Job drawing, mm, ordinate dimensions from the low corner. One solid piece. Give positions to 0.01 mm unless a question says otherwise; leave off trailing zeros. Order: outer loops, then holes, each group sorted by start corner. A loop starts at its lowest first (then second) coordinate and runs counter-clockwise, first axis right, second up. Notation, with made-up numbers: (6, 67) -> (13, 67) arc R9 ccw to (13, 75) -> close; hole circle Ø10 at (88, 29). An arc over 180 degrees is marked (long way). Use CSV: the item, a comma, the result in double quotes. Start each with the question number.
1. Cut at B-B on z = 63.5. List the corners of the cut face in (x, y) (3 decimals).
2. Cut at A-A on x = 63.5. List the corners of the cut face in (y, z) (3 decimals), then the cut area to 3 significant figures.
3. Cut at D-D on y = 1.55. List the corners of the cut face in (x, z) (3 decimals), then the cut area to 3 significant figures.
4. Drop a flat-ended pin along its axis: pin 1 (2.5 mm diameter, centred on x = 44.45, z = 31.75, fed in from +Y). Give the stop position or say it passes through.
5. Wall check: line 1 (X direction, y = 2.05, z = 95.25) (3 decimals); line 2 (Z direction, x = 76.5, y = 1.5); line 3 (Z direction, x = 71, y = 1). Give the ranges that are in metal, low to high. Write a range as from..to.
6. Cut at C-C on z = 95.25. List the corners of the cut face in (x, y) (3 decimals), then the cut area to 3 significant figures.
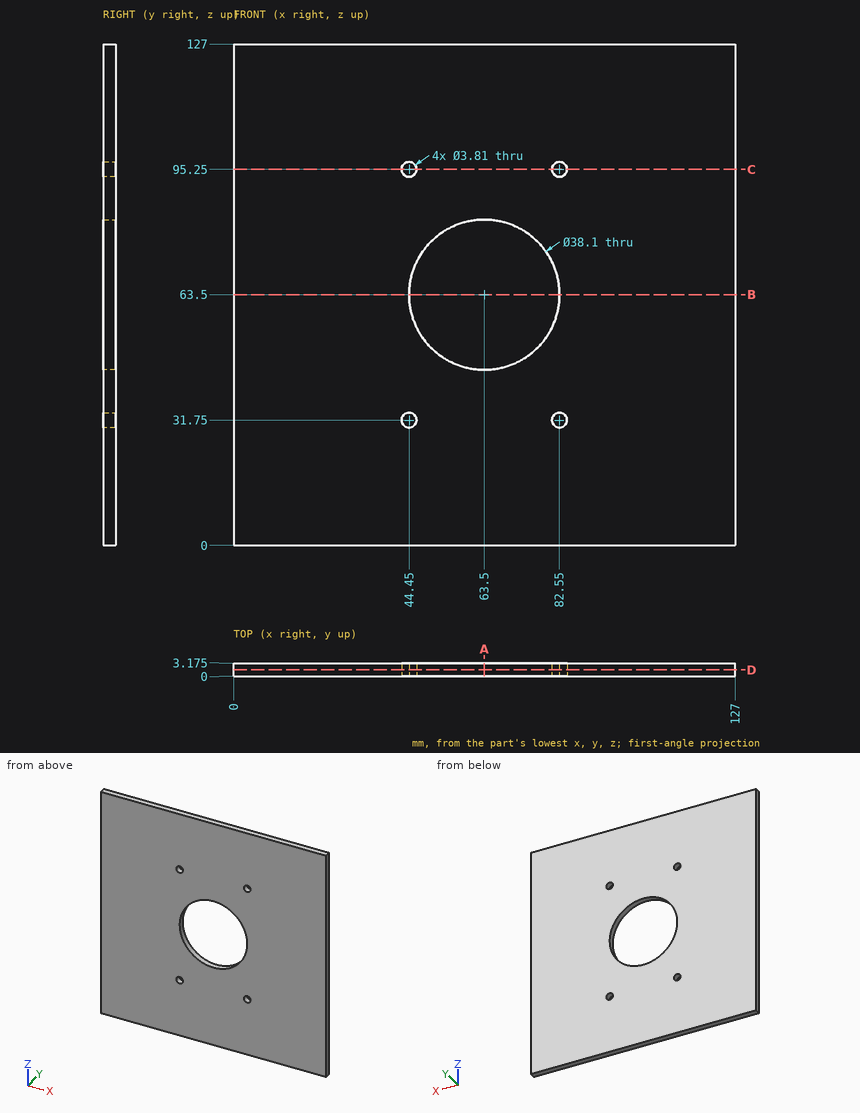
Verdict:
1,outline,"(0, 0) -> (44.45, 0) -> (44.45, 3.175) -> (0, 3.175) -> close; (82.55, 0) -> (127, 0) -> (127, 3.175) -> (82.55, 3.175) -> close"
2,outline,"(0, 0) -> (3.175, 0) -> (3.175, 44.45) -> (0, 44.45) -> close; (0, 82.55) -> (3.175, 82.55) -> (3.175, 127) -> (0, 127) -> close"
2,area,"282 mm^2"
3,outline,"(0, 0) -> (127, 0) -> (127, 127) -> (0, 127) -> close; hole circle Ø3.81 at (44.45, 31.75); hole circle Ø3.81 at (44.45, 95.25); hole circle Ø38.1 at (63.5, 63.5); hole circle Ø3.81 at (82.55, 31.75); hole circle Ø3.81 at (82.55, 95.25)"
3,area,"14,900 mm^2"
4,pin 1,"through"
5,line 1,"0..42.545, 46.355..80.645, 84.455..127"
5,line 2,"0..49.58, 77.42..127"
5,line 3,"0..45.99, 81.01..127"
6,outline,"(0, 0) -> (42.545, 0) -> (42.545, 3.175) -> (0, 3.175) -> close; (46.355, 0) -> (80.645, 0) -> (80.645, 3.175) -> (46.355, 3.175) -> close; (84.455, 0) -> (127, 0) -> (127, 3.175) -> (84.455, 3.175) -> close"
6,area,"379 mm^2"
